Geometry: final body of the model. Coordinates: model frame, mm. A direction names the side the tool comes from. Give positions to 0.01 mm unless a question says otherwise; leave off trailing zeros. Write each loop counter-clockwise with the first axis right and the second up, starting at its lowest first coordinate (ties: lowest second). Pieces come first, ordered by that corner, then holes. Notation, with made-up numbers: M -29.75,-0.5 L -25.75,-0.5 A24 ccw -25.75,21.5 Z; hole C 69,31 d2. An arc over 180 degrees is marked long. Use a Markdown table: item, result. Add a question column.
1) Section C-C on x = 23. Return the cut outline in (y, z), then the cut area to 3 significant figures.
2) Line query: line 1 (Y direction, x = 11.5, z = -2); line 2 (X direction, y = -20, z = 19); line 3 (Y direction, x = 15, z = 3). Output: solid intervals per line, ascending.
3) Draft query along Y for faces 1 (the cylindrical face through (30.222, -35.706, 7.929)), 2 (the flat face through (16.828, 0, 0)), 3 (the flat face through (8.255, 3, 3)). Return one class per face: +Y half, -Y half, draft (parallel to the pull), parting line (faces both ways), or undercut.
4) Set-up query: faces 4 (the flat face through (26.25, -15, -15)), 5 (the flat face through (34.25, 0, 0)). Return all of +Z, -Z, +X, -X, +Y, -Y with unobstructed straight access to the full face (end or side cutting, diameter ignored); none if empty.
5) Section B-B on x = 15.75. Return the cut outline in (y, z), then the cut area to 3 significant figures.
6) Pin query (flat end, axial travel): pin 1 (2 mm diameter, centred on x = 26.5, y = 21, fed in from -Z); pin 2 (1 mm diameter, centred on x = 31, y = -5.5, fed in from -Z); pin 3 (1.5 mm diameter, centred on x = 22, y = -16.5, fed in from +Z). Return the tip coordinate at first contact, or that it passes through.
7) Section D-D on x = 31.25. Return the cut outline in (y, z), then the cut area to 3 significant figures.
```python
from build123d import *

# Parameters (mm, degrees)
SKETCH1_W           = 17.995
SKETCH1_H           = 18.542
SKETCH2_R           = 3.71475
CUT_EXTRUDE1_DEPTH  = 8.5725
CUT_EXTRUDE1_TAPER  = 3
SKETCH3_R           = 36.576
BOSS_EXTRUDE1_DEPTH = 8
FILLET1_R           = 2
SKETCH4_R           = 18.542
SKETCH4_R_2         = 12.7
CUT_EXTRUDE2_DEPTH  = 2
FILLET2_R           = 5


with BuildPart() as part:
    # Sketch1 → Revolve1 (revolve)
    with BuildSketch(Plane.XY):
        with Locations((17.2525, 9.271)):
            Rectangle(SKETCH1_W, SKETCH1_H)
    revolve(axis=Axis((8.255, 0, 0), (1, 0, 0)))

    # Sketch2 → Cut-Extrude1 (cut)
    with BuildSketch(Plane.ZY.offset(-8.255)):
        Circle(SKETCH2_R)
    extrude(amount=-CUT_EXTRUDE1_DEPTH, taper=CUT_EXTRUDE1_TAPER, mode=Mode.SUBTRACT)

    # Sketch3 → Boss-Extrude1 (add)
    with BuildSketch(Plane(origin=(26.25, 0, 0), x_dir=(0, 0, -1), z_dir=(1, 0, 0))):
        Circle(SKETCH3_R)
    extrude(amount=BOSS_EXTRUDE1_DEPTH)

    # Fillet1
    fillet1_edges = [part.edges().sort_by_distance(p)[0] for p in [
        (26.25, -18.542, 0),
        (26.25, 0, 36.576),
        (34.25, 0, 36.576),
    ]]
    fillet(fillet1_edges, radius=FILLET1_R)

    # Sketch4 → Cut-Extrude2 (cut)
    with BuildSketch(Plane.ZY.offset(-8.255)):
        Circle(SKETCH4_R)
        Circle(SKETCH4_R_2, mode=Mode.SUBTRACT)
    extrude(amount=-CUT_EXTRUDE2_DEPTH, mode=Mode.SUBTRACT)

    # Sketch5 → Revolve2 (revolve)
    with BuildSketch(Plane(origin=(0, 0, 0), x_dir=(1, 0, 0), z_dir=(0, 1, 0))):
        Polygon((8.255, -12.7), (10.255, -18.542), (10.255, -12.7), align=None)
    revolve(axis=Axis((0, 0, 0), (1, 0, 0)))

    # Fillet2
    fillet2_edges = [part.edges().sort_by_distance(p)[0] for p in [
        (8.255, 0, -12.7),
    ]]
    fillet(fillet2_edges, radius=FILLET2_R)


solid = part.part
```
Found:
| question | item | result |
|---|---|---|
| 1 | outline | C 0,0 d37.08 |
| 1 | area | 1,080 mm² |
| 2 | line 1 | -18.43 to -2.93, 2.93 to 18.43 |
| 2 | line 2 | 26.25 to 34.25 |
| 2 | line 3 | -18.3 to -1.52, 1.52 to 18.3 |
| 3 | face 1 | parting line |
| 3 | face 2 | undercut |
| 3 | face 3 | draft |
| 4 | face 4 | -X |
| 4 | face 5 | +Z, -Z, +X, +Y, -Y |
| 5 | outline | C 0,0 d37.08; hole C 0,0 d6.64 |
| 5 | area | 1,050 mm² |
| 6 | pin 1 | z = -30.08 |
| 6 | pin 2 | z = -36.23 |
| 6 | pin 3 | z = 9.78 |
| 7 | outline | C 0,0 d73.15 |
| 7 | area | 4,200 mm² |
